```python
from build123d import *

# Parameters (mm, degrees)
BOSS_EXTRUDE9_DEPTH      = 5.6
BOSS_EXTRUDE9_DEPTH_BACK = 2
SKETCH16_W               = 8
SKETCH16_H               = 3.5
BOSS_EXTRUDE11_DEPTH     = 8
CHAMFER2_SIZE            = 1.5
SKETCH17_W               = 3.94
SKETCH17_H               = 8
BOSS_EXTRUDE12_DEPTH     = 6.3
CUT_EXTRUDE2_START       = -5.6
CUT_EXTRUDE2_DEPTH       = 3.6
SKETCH21_R               = 1.5
BOSS_EXTRUDE14_DEPTH     = 3.6
CHAMFER4_SIZE            = 1
CUT_EXTRUDE3_DEPTH       = 3.6
SPLIT1_START             = -2
SPLIT1_DEPTH             = 7.6
SKETCH22_R               = 5
BOSS_EXTRUDE15_DEPTH     = 2
SKETCH23_R               = 3
BOSS_EXTRUDE16_DEPTH     = 8
CUT_EXTRUDE4_DEPTH       = 32.952026383
CUT_EXTRUDE4_DEPTH_BACK  = 8
SKETCH24_R               = 2
CHAMFER5_SIZE            = 0.5
CHAMFER5_SIZE2           = 1
SKETCH25_W               = 1.53
SKETCH25_H               = 2
BOSS_EXTRUDE17_DEPTH     = 8
CHAMFER6_SIZE            = 0.5


# Read off the part's stored shape, not the designer's step: Split1
with BuildPart() as part:
    # Sketch14 → Boss-Extrude9 (new, two sides: drawn at the far end of the back side and taken through both)
    with BuildSketch(Plane(origin=(0, 0, 0), x_dir=(1, 0, 0), z_dir=(0, 1, 0)).offset(-BOSS_EXTRUDE9_DEPTH_BACK)):
        with BuildLine():
            Line((-4.172171186, -20.619968889), (-4.172171186, -25.619968889))
            Line((-4.172171186, -25.619968889), (7.827828814, -25.619968889))
            Line((7.827828814, -25.619968889), (7.827828814, -20.619968889))
            ThreePointArc((7.827828814, -20.619968889), (1.827828814, -14.619968889), (-4.172171186, -20.619968889))
        make_face()
    extrude(amount=BOSS_EXTRUDE9_DEPTH + BOSS_EXTRUDE9_DEPTH_BACK)

    # Sketch16 → Boss-Extrude11 (add)
    with BuildSketch(Plane.XY.offset(25.619968889)):
        with Locations((1.827828814, 1.75)):
            Rectangle(SKETCH16_W, SKETCH16_H)
    extrude(amount=BOSS_EXTRUDE11_DEPTH)

    # Chamfer2
    chamfer2_edges = [part.edges().sort_by_distance(p)[0] for p in [
        (1.827828814, -2, 14.619968889),
        (7.827828814, 5.6, 23.119968889),
        (1.827828814, 5.6, 14.619968889),
        (-4.172171186, -2, 23.119968889),
        (-4.172171186, 5.6, 23.119968889),
        (7.827828814, -2, 23.119968889),
    ]]
    chamfer(chamfer2_edges, length=CHAMFER2_SIZE)

    # Sketch17 → Boss-Extrude12 (add)
    with BuildSketch(Plane.XZ.offset(2)):
        with Locations((1.827828814, 21.619968889)):
            Rectangle(SKETCH17_W, SKETCH17_H)
    extrude(amount=BOSS_EXTRUDE12_DEPTH)

    # Sketch20 → Cut-Extrude2 (cut)
    with BuildSketch(Plane(origin=(0, 5.6, 0), x_dir=(1, 0, 0), z_dir=(0, 1, 0)).offset(CUT_EXTRUDE2_START)):
        with BuildLine():
            Line((7.827828814, -20.619968889), (-4.172171186, -20.619968889))
            ThreePointArc((-4.172171186, -20.619968889), (1.827828814, -14.619968889), (7.827828814, -20.619968889))
        make_face()
    extrude(amount=CUT_EXTRUDE2_DEPTH, mode=Mode.SUBTRACT)

    # Sketch21 → Boss-Extrude14 (add)
    with BuildSketch(Plane(origin=(0, 0, 0), x_dir=(1, 0, 0), z_dir=(0, 1, 0))):
        with BuildLine():
            ThreePointArc((7.827828814, -20.619968889), (7.63955943, -19.128732072), (7.086566399, -17.731080001))
            ThreePointArc((7.086566399, -17.731080001), (6.279209969, -19.350325806), (4.990106474, -20.619968889))
            Line((4.990106474, -20.619968889), (7.827828814, -20.619968889))
        make_face()
        with BuildLine():
            ThreePointArc((-1.334448847, -20.619968889), (-2.623552342, -19.350325806), (-3.430908771, -17.731080001))
            ThreePointArc((-3.430908771, -17.731080001), (-3.983901803, -19.128732072), (-4.172171186, -20.619968889))
            Line((-4.172171186, -20.619968889), (-1.334448847, -20.619968889))
        make_face()
        with Locations(Location((1.827828814, -16.119968889, 0), (0, 0, 90.000763944))):
            Circle(SKETCH21_R)
    extrude(amount=BOSS_EXTRUDE14_DEPTH)

    # Chamfer4
    # the kernel refuses this chamfer: 1 mm, written as the material it adds along each edge
    with BuildSketch(Plane(origin=(1.827828814, 3.6, 16.119968889), x_dir=(-1.3333338100422289e-05, 0, -0.999999999911111), z_dir=(0.999999999911111, 0, -1.3333338100422289e-05))) as chamfer4_piece_1_section:
        Polygon((1.5, -CHAMFER4_SIZE), (1.5 + CHAMFER4_SIZE, 0), (1.5, 0), align=None)
    chamfer4_piece_1 = revolve(axis=Axis((1.827828814, 3.6, 16.119968889), (0, 1, 0)), mode=Mode.PRIVATE)
    chamfer4_piece_1 = chamfer4_piece_1 & Plane(origin=(1.827828814, 3.111670507, 20.619968889), x_dir=(1, 0, 0), z_dir=(0, -1, 0)) * Cylinder(6, 10, mode=Mode.PRIVATE)
    add(chamfer4_piece_1)
    with BuildSketch(Plane(origin=(1.827828814, 0, 16.119968889), x_dir=(-1.3333338100422289e-05, 0, -0.999999999911111), z_dir=(0.999999999911111, 0, -1.3333338100422289e-05))) as chamfer4_piece_2_section:
        Polygon((1.5 + CHAMFER4_SIZE, 0), (1.5, CHAMFER4_SIZE), (1.5, 0), align=None)
    chamfer4_piece_2 = revolve(axis=Axis((1.827828814, 0, 16.119968889), (0, 1, 0)), mode=Mode.PRIVATE)
    chamfer4_piece_2 = chamfer4_piece_2 & Plane(origin=(1.827828814, 0.488329493, 20.619968889), x_dir=(1, 0, 0), z_dir=(0, -1, 0)) * Cylinder(6, 10, mode=Mode.PRIVATE)
    add(chamfer4_piece_2)

    # Sketch21<3> → Cut-Extrude3 (cut)
    with BuildSketch(Plane(origin=(0, 0, 0), x_dir=(1, 0, 0), z_dir=(0, 1, 0))):
        with BuildLine():
            Line((4.990106474, -20.619968889), (-1.334448847, -20.619968889))
            ThreePointArc((-1.334448847, -20.619968889), (1.827828814, -21.619968889), (4.990106474, -20.619968889))
        make_face()
    extrude(amount=CUT_EXTRUDE3_DEPTH, mode=Mode.SUBTRACT)

    # Split1 outline → Split1 (cut)
    with BuildSketch(Plane(origin=(0, 0, 0), x_dir=(1, 0, 0), z_dir=(0, 1, 0)).offset(SPLIT1_START)):
        with BuildLine():
            Line((7.827828814, -25.619968889), (7.827828814, -20.619968889))
            ThreePointArc((7.827828814, -20.619968889), (1.827828814, -14.619968889), (-4.172171186, -20.619968889))
            Line((-4.172171186, -20.619968889), (-4.172171186, -25.619968889))
            Line((-4.172171186, -25.619968889), (-2.172171186, -25.619968889))
            Line((-2.172171186, -25.619968889), (-2.172171186, -33.619968889))
            Line((-2.172171186, -33.619968889), (5.827828814, -33.619968889))
            Line((5.827828814, -33.619968889), (5.827828814, -25.619968889))
            Line((5.827828814, -25.619968889), (7.827828814, -25.619968889))
        make_face()
    extrude(amount=SPLIT1_DEPTH, mode=Mode.SUBTRACT)

    # Sketch22 → Boss-Extrude15 (add)
    with BuildSketch(Plane(origin=(0, -2, 0), x_dir=(1, 0, 0), z_dir=(0, 1, 0))):
        with Locations(Location((1.827828814, -21.619968889, 0), (0, 0, 270))):
            Circle(SKETCH22_R)
    extrude(amount=BOSS_EXTRUDE15_DEPTH)

    # Sketch23 → Boss-Extrude16 (add)
    with BuildSketch(Plane(origin=(0, 0, 0), x_dir=(1, 0, 0), z_dir=(0, 1, 0))):
        with Locations(Location((1.827828814, -21.619968889, 0), (0, 0, 270))):
            Circle(SKETCH23_R)
    extrude(amount=BOSS_EXTRUDE16_DEPTH)

    # Sketch24 → Cut-Extrude4 (cut, two sides: drawn at the far end of the back side and taken through both)
    with BuildSketch(Plane(origin=(0, 8, 0), x_dir=(1, 0, 0), z_dir=(0, 1, 0)).offset(-CUT_EXTRUDE4_DEPTH_BACK)):
        with Locations(Location((1.827828814, -21.619968889, 0), (0, 0, 270))):
            Circle(SKETCH24_R)
    extrude(amount=CUT_EXTRUDE4_DEPTH + CUT_EXTRUDE4_DEPTH_BACK, mode=Mode.SUBTRACT)

    # Chamfer5
    chamfer5_edges = [part.edges().sort_by_distance(p)[0] for p in [
        (1.827828814, 8, 19.619968889),
    ]]
    chamfer5_side = [part.faces().sort_by_distance(p)[0] for p in [
        (1.827828814, 8, 18.704821703),
    ]]
    chamfer(chamfer5_edges, length=CHAMFER5_SIZE, length2=CHAMFER5_SIZE2, reference=chamfer5_side[0])

    # Sketch25 → Boss-Extrude17 (add)
    with BuildSketch(Plane.XY.offset(25.619968889)):
        Polygon((3.797828814, -4.5), (3.797828814, -6.3), (5.327828814, -6.3), align=None)
        with Locations((4.562828814, -7.3)):
            Rectangle(SKETCH25_W, SKETCH25_H)
        with Locations((-0.907171186, -7.3)):
            Rectangle(SKETCH25_W, SKETCH25_H)
        Polygon((-0.142171186, -4.5), (-1.672171186, -6.3), (-0.142171186, -6.3), align=None)
    extrude(amount=-BOSS_EXTRUDE17_DEPTH)

    # Chamfer6
    chamfer6_edges = [part.edges().sort_by_distance(p)[0] for p in [
        (3.797828814, -3.25, 17.619968889),
        (-0.142171186, -3.25, 17.619968889),
        (3.797828814, -3.25, 25.619968889),
        (-0.142171186, -3.25, 25.619968889),
        (5.327828814, -7.3, 17.619968889),
        (5.327828814, -7.3, 25.619968889),
        (5.327828814, -8.3, 21.619968889),
        (4.562828814, -5.4, 25.619968889),
        (4.562828814, -5.4, 17.619968889),
        (-1.672171186, -8.3, 21.619968889),
        (-0.907171186, -5.4, 17.619968889),
        (-0.907171186, -5.4, 25.619968889),
        (-1.672171186, -7.3, 25.619968889),
        (-1.672171186, -7.3, 17.619968889),
        (1.827828814, -8.3, 25.619968889),
        (1.827828814, -8.3, 17.619968889),
    ]]
    chamfer(chamfer6_edges, length=CHAMFER6_SIZE)


solid = part.part
```
The listing builds one solid part. Answer for the finished solid, in the listing's coordinates (mm). A direction names the side the tool comes from. Give positions to 0.01 mm unless a question says otherwise; leave off trailing zeros. Order: outer loops, then holes, each group sorted by start corner. A loop starts at its lowest first (then second) coordinate and runs counter-clockwise, first axis right, second up. Notation, with made-up numbers: (-14, -36) -> (13, -36) arc R22 cw to (13, 3) -> close; hole circle Ø4 at (25.5, 12.25). An arc over 180 degrees is marked (long way). Answer as CSV lines item,"result". Start each with the question number.
Q1. A cutting plane is placed at A-A (y = -3.5). Determine the outline of the cut face in (x, z), then the cut area to 3 significant figures.
Q2. Given pin 1 (5 mm diameter, centred on x = 1.5, y = 5.5, fed in from +Z); pin 2 (0.5 mm diameter, centred on y = -7, z = 20.5, fed in from +X); pin 3 (6 mm diameter, centred on x = 5.5, y = -5, fed in from -Z), each flat-ended and moving along its own axis, determine where each tip first touches the part or whether it passes through.
Q3. Find the intervals of material crossed by L1, parallel to Y at x = -0.5, z = 21.75; L2, parallel to Y at x = 0.25, z = 19; L3, parallel to Y at x = -1, z = 21.25, in increasing order.
Q4. A cutting plane is placed at B-B (y = 5.75). Determine the outline of the cut face in (x, z).
Q5. A cutting plane is placed at D-D (y = -0.5). Determine the outline of the cut face in (x, z).
Q6. Determine the mould class of faces 1 (the flat face through (-1.4, 0, 21.5)), 2 (the flat face through (2, -6, 17.62)), 3 (the flat face through (4.327, -5.503, 17.873)) for opening direction Y: pulls with the +Y half, pulls with the -Y half, needs draft (parallel to the pull), parting line crosses it, or undercut.
Q7. Which of the six approach directions +Z, -Z, +X, -X, +Y, -Y give full straight-line access (tool end or side, diameter ignored) to faces 4 (the flat face through (-0.643, -5.481, 25.373)), 5 (the flat face through (-0.9, -5.39, 21.67)), 6 (the flat face through (3.798, -3, 22)), 7 (the flat face through (-1.672, -7, 22)), 8 (the flat face through (4.322, -5.508, 25.373))?
Q8. A cutting plane is placed at C-C (x = 6). Determine the outline of the cut face in (y, z), then the cut area to 3 significant figures.
Results found:
1,outline,"(-0.14, 18.12) -> (0.36, 17.62) -> (3.3, 17.62) -> (3.8, 18.12) -> (3.8, 25.12) -> (3.3, 25.62) -> (0.36, 25.62) -> (-0.14, 25.12) -> close"
1,area,"31.0 mm2"
2,pin 1,"z = 24.62"
2,pin 2,"x = 5.33"
2,pin 3,"z = 17.62"
3,L1,"-8.3 to -4.92, -2 to 7.66"
3,L2,"-8.3 to 0"
3,L3,"-8.3 to -5.51, -2 to 8"
4,outline,"circle Ø6 at (1.83, 21.62); hole circle Ø4 at (1.83, 21.62)"
5,outline,"circle Ø10 at (1.83, 21.62)"
6,face 1,"pulls with the +Y half"
6,face 2,"needs draft"
6,face 3,"undercut"
7,face 4,"+Z, -X"
7,face 5,"+Z, -Z, -X"
7,face 6,"+Z, -Z, +X"
7,face 7,"+Z, -Z, -X, -Y"
7,face 8,"+Z, +X"
8,outline,"(-2, 18.86) -> (0, 18.86) -> (0, 24.38) -> (-2, 24.38) -> close"
8,area,"11.0 mm2"
